Design review of the part built by this model. Coordinates are the model's own, in mm. A direction names the side the tool comes from. Coordinates: 2 decimals unless noted, no trailing zeros. Loops run counter-clockwise (first coordinate to the right, second up) from the corner with the lowest first, then second, coordinate; pieces in that order, holes last. Notation, with made-up numbers: (29.5, 59.5) - (51.5, 59.5) arc R12 cw to (51.5, 63.5) - close; hole circle Ø9 at (-25, 53). An arc over 180 degrees is marked (long way). Answer in a Markdown table with one row per item. Add a question column.
(1) We need section B-B, the plane y = -3. Write out the cut boundary in (x, z).
(2) We need section D-D, the plane x = -2.75. Write out the cut boundary in (y, z).
(3) To check wall thickness, follow L1, parallel to X at y = 11.5, z = 7.5; L2, parallel to Y at x = 0, z = 7; L3, parallel to Y at x = -5.25, z = 5.75. State the ranges of each line that lie inside material, in increasing order. Write a range as [from, to].
(4) The part is to be moulded in two halves that separate along Z. For faces 3 (the face through (0.22, -14.26, 9.95)), 4 (the face through (6.9, 14.43, 5.92)), 5 (the face through (0, 0, 10)), say which applies: released by +Z, released by -Z, zero draft, split by the parting line, or undercut.
(5) Clearance check with a flat-ended pin moving along its axis: pin 1 (6 mm diameter, centred on x = -0.5, y = 5, fed in from -Z). State where the tip first meets the part, or that it passes through.
(6) We need section C-C, the plane z = 5. Write out the cut boundary in (x, y).
(7) We need section A-A, the plane x = 0. Write out the cut boundary in (y, z), plus the area to 3 significant figures.
(8) For faces 1 (the face through (6, 0, 5)), 2 (the face through (6.9, -14.43, 6.08)), list the 3-axis set-ups (+Z, -Z, +X, -X, +Y, -Y) from which the entire face can be reached by the end or side of a thin tool; tool diameter is ignored.
from build123d import *

# Parameters (mm, degrees)
SKETCH1_W                       = 15
SKETCH1_H                       = 30
SKETCH1_W_2                     = 12
SKETCH1_H_2                     = 27
BOSS_EXTRUDE1_DEPTH             = 10
BOSS_EXTRUDE2_REACH             = 33.121
SKETCH2_W                       = 15
SKETCH2_H                       = 2
BOSS_EXTRUDE2_DIRECTION_2_REACH = 33.121
SKETCH3_R                       = 4.953
CUT_EXTRUDE2_DEPTH              = 10
FILLET1_R                       = 2


with BuildPart() as part:
    # Sketch1 → Boss-Extrude1 (new body)
    with BuildSketch(Plane.XY):
        Rectangle(SKETCH1_W, SKETCH1_H)
        Rectangle(SKETCH1_W_2, SKETCH1_H_2, mode=Mode.SUBTRACT)
    extrude(amount=BOSS_EXTRUDE1_DEPTH)

    # Boss-Extrude2: up to this face of the body (flat: up to its plane)
    boss_extrude2_end = Plane(part.part.faces().sort_by_distance((0, 15, 5))[0])
    # Sketch2 → Boss-Extrude2 (add, up to the picked face)
    with BuildSketch(Plane(origin=(0, -13.5, 0), x_dir=(1, 0, 0), z_dir=(0, 1, 0)), mode=Mode.PRIVATE) as boss_extrude2_sk1:
        with Locations((0, -11)):
            Rectangle(SKETCH2_W, SKETCH2_H)
    boss_extrude2_tool1 = split(extrude(boss_extrude2_sk1.sketch, amount=BOSS_EXTRUDE2_REACH, mode=Mode.PRIVATE), bisect_by=boss_extrude2_end, keep=Keep.BOTH, mode=Mode.PRIVATE)
    add(boss_extrude2_tool1.solids().sort_by(Axis((0, -13.5, 11), (0, 1, 0)))[0])

    # Boss-Extrude2 direction 2: up to this face of the body (flat: up to its plane)
    boss_extrude2_direction_2_end = Plane(part.part.faces().sort_by_distance((0, -15, 5))[0])
    # Sketch2 → Boss-Extrude2 direction 2 (add, up to the picked face)
    with BuildSketch(Plane(origin=(0, -13.5, 0), x_dir=(1, 0, 0), z_dir=(0, 1, 0)), mode=Mode.PRIVATE) as boss_extrude2_direction_2_sk1:
        with Locations((0, -11)):
            Rectangle(SKETCH2_W, SKETCH2_H)
    boss_extrude2_direction_2_tool1 = split(extrude(boss_extrude2_direction_2_sk1.sketch, amount=-BOSS_EXTRUDE2_DIRECTION_2_REACH, mode=Mode.PRIVATE), bisect_by=boss_extrude2_direction_2_end, keep=Keep.BOTH, mode=Mode.PRIVATE)
    add(boss_extrude2_direction_2_tool1.solids().sort_by(Axis((0, -13.5, 11), (0, -1, 0)))[0])

    # Sketch3 → Cut-Extrude2 (cut)
    with BuildSketch(Plane.XZ.offset(15)):
        with Locations(Location((0, 5, 0), (0, 0, 270))):
            Circle(SKETCH3_R)
    extrude(amount=-CUT_EXTRUDE2_DEPTH, mode=Mode.SUBTRACT)

    # Fillet1
    fillet1_edges = [part.edges().sort_by_distance(p)[0] for p in [
        (-7.5, 15, 6),
        (7.5, 15, 6),
        (7.5, -15, 6),
        (-7.5, -15, 6),
    ]]
    fillet(fillet1_edges, radius=FILLET1_R)


solid = part.part
Responses:
| question | item | result |
|---|---|---|
| 1 | outline | (-7.5, 0) - (-6, 0) - (-6, 10) - (6, 10) - (6, 0) - (7.5, 0) - (7.5, 12) - (-7.5, 12) - close |
| 2 | outline | (-15, 0) - (-13.5, 0) - (-13.5, 0.88) - (-15, 0.88) - close; (-15, 9.12) - (-13.5, 9.12) - (-13.5, 10) - (13.5, 10) - (13.5, 0) - (15, 0) - (15, 12) - (-15, 12) - close |
| 3 | L1 | x = [-7.5, -6], [6, 7.5] |
| 3 | L2 | y = [13.5, 15] |
| 3 | L3 | y = [-15, -13.5], [13.5, 15] |
| 4 | face 3 | undercut |
| 4 | face 4 | zero draft |
| 4 | face 5 | released by -Z |
| 5 | pin 1 | stops at z = 10 |
| 6 | outline | (-7.5, -13) arc R2 ccw to (-5.5, -15) - (-4.95, -15) - (-4.95, -13.5) - (-6, -13.5) - (-6, 13.5) - (6, 13.5) - (6, -13.5) - (4.95, -13.5) - (4.95, -15) - (5.5, -15) arc R2 ccw to (7.5, -13) - (7.5, 13) arc R2 ccw to (5.5, 15) - (-5.5, 15) arc R2 ccw to (-7.5, 13) - close |
| 7 | outline | (-15, 0) - (-13.5, 0) - (-13.5, 0.05) - (-15, 0.05) - close; (-15, 9.95) - (-13.5, 9.95) - (-13.5, 10) - (13.5, 10) - (13.5, 0) - (15, 0) - (15, 12) - (-15, 12) - close |
| 7 | area | 75.1 mm2 |
| 8 | face 1 | -Z |
| 8 | face 2 | +Z, -Z, +X, -Y |
